Work out the finished part from the listing and answer in its coordinate system (mm). Round coordinates to 2 decimals unless told otherwise and drop trailing zeros. Order: outer loops, then holes, each group sorted by start corner. A loop starts at its lowest first (then second) coordinate and runs counter-clockwise, first axis right, second up. Notation, with made-up numbers: (38.25, -34.75) - (45.25, -34.75) arc R24 ccw to (45.25, -20.75) - close; hole circle Ø7 at (56.25, 46). An arc over 180 degrees is marked (long way). Answer in a Markdown table with one row per item.
from build123d import *

# Parameters (mm, degrees)
PAD_DEPTH = 10


with BuildPart() as part:
    # Sketch → Pad (new body, symmetric)
    with BuildSketch(Plane.XZ):
        with BuildLine():
            ThreePointArc((-6.03596, 0.051174), (-7.12656, 1.0918), (-8.21716, 0.051174))
            ThreePointArc((-9.6, 0.0836), (-8.924417, -0.60801), (-8.21716, 0.051174))
            Line((-9.6, 0.0836), (-10, 0.0836))
            ThreePointArc((-10, 0.0836), (-8.933794, -1.0079), (-7.8176, 0.032426))
            ThreePointArc((-6.43552, 0.032426), (-7.12656, 0.6918), (-7.8176, 0.032426))
            ThreePointArc((-6.43552, 0.032426), (-5.34492, -1.0082), (-4.25432, 0.032426))
            ThreePointArc((-2.87224, 0.032426), (-3.56328, 0.6918), (-4.25432, 0.032426))
            ThreePointArc((-2.87224, 0.032426), (-1.78164, -1.0082), (-0.69104, 0.032426))
            ThreePointArc((0.69104, 0.032426), (0, 0.6918), (-0.69104, 0.032426))
            ThreePointArc((0.69104, 0.032426), (1.78164, -1.0082), (2.87224, 0.032426))
            ThreePointArc((4.25432, 0.032426), (3.56328, 0.6918), (2.87224, 0.032426))
            ThreePointArc((4.25432, 0.032426), (5.34492, -1.0082), (6.43552, 0.032426))
            ThreePointArc((7.8176, 0.032426), (7.12656, 0.6918), (6.43552, 0.032426))
            ThreePointArc((7.8176, 0.032426), (8.933794, -1.0079), (10, 0.0836))
            Line((9.6, 0.0836), (10, 0.0836))
            ThreePointArc((8.21716, 0.051174), (8.924417, -0.60801), (9.6, 0.0836))
            ThreePointArc((8.21716, 0.051174), (7.12656, 1.0918), (6.03596, 0.051174))
            ThreePointArc((4.65388, 0.051174), (5.34492, -0.6082), (6.03596, 0.051174))
            ThreePointArc((4.65388, 0.051174), (3.56328, 1.0918), (2.47268, 0.051174))
            ThreePointArc((1.0906, 0.051174), (1.78164, -0.6082), (2.47268, 0.051174))
            ThreePointArc((1.0906, 0.051174), (0, 1.0918), (-1.0906, 0.051174))
            ThreePointArc((-2.47268, 0.051174), (-1.78164, -0.6082), (-1.0906, 0.051174))
            ThreePointArc((-2.47268, 0.051174), (-3.56328, 1.0918), (-4.65388, 0.051174))
            ThreePointArc((-6.03596, 0.051174), (-5.34492, -0.6082), (-4.65388, 0.051174))
        make_face()
    extrude(amount=PAD_DEPTH, both=True)


solid = part.part
1) Find section C-C, the plane x = 0. Give the vertices of the cut face in (y, z), then the cut area to 3 significant figures.
Filled in:
| item | result |
|---|---|
| outline | (-10, 0.69) - (10, 0.69) - (10, 1.09) - (-10, 1.09) - close |
| area | 8.00 mm^2 |
2) Find the intervals of material crossed by probe 1 along X at (y, z) = (-9, -0.65); probe 2 along X at (y, z) = (8, -0.9); probe 3 along X at (y, z) = (-3.25, 0.95), in increasing order. Write a range as from..to.
Filled in:
| item | result |
|---|---|
| probe 1 | x = -9.72..-8.1, -6.15..-4.54, -2.59..-0.97, 0.97..2.59, 4.54..6.15, 8.1..9.72 |
| probe 2 | x = -9.38..-8.43, -5.82..-4.87, -2.26..-1.31, 1.31..2.26, 4.87..5.82, 8.43..9.38 |
| probe 3 | x = -7.66..-6.59, -4.1..-3.03, -0.54..0.54, 3.03..4.1, 6.59..7.66 |
3) The mould has two halves that part along X. Classify faces 1 (the face through (-3.55, -0.14, 0.69)), 2 (the face through (-0.8, -10, 0.4)), 3 (the face through (-4, 0, 1)): released by +X, released by -X, zero draft, split by the parting line, or undercut.
Filled in:
| item | result |
|---|---|
| face 1 | undercut |
| face 2 | zero draft |
| face 3 | undercut |
4) This flat-tipped pin is pushed along its axis until it touches: pin 1 (2 mm diameter, centred on x = 5.5, y = -0.5, fed in from +Z). Where does it stop, or does it pass through?
Filled in:
| item | result |
|---|---|
| pin 1 | stops at z = 0.89 |
5) Find section B-B, the plane z = 0.45. Give the number of separate pieces and of enclosed holes in the cut face, then the cut area to 3 significant figures.
Filled in:
| item | result |
|---|---|
| separate pieces | 10 |
| enclosed holes | 0 |
| area | 93.9 mm^2 |
6) Find section D-D, the plane x = 7.25. Give the vertices of the cut face in (y, z), then the cut area to 3 significant figures.
Filled in:
| item | result |
|---|---|
| outline | (-10, 0.68) - (10, 0.68) - (10, 1.08) - (-10, 1.08) - close |
| area | 8.08 mm^2 |
